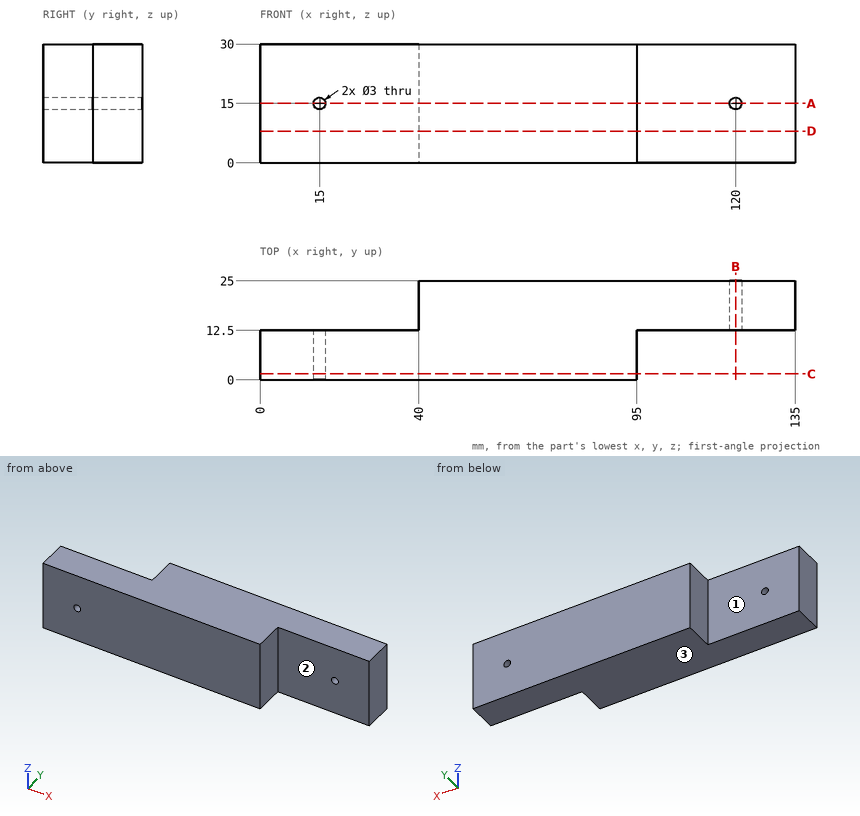
Check sheet for the drawn part. Datum: minimum x, y, z corner. Units: mm. A direction names the side the tool comes from. Round coordinates to 2 decimals unless told otherwise and drop trailing zeros. Order: outer loops, then holes, each group sorted by start corner. A loop starts at its lowest first (then second) coordinate and runs counter-clockwise, first axis right, second up.
1) Tool access check on the marked faces 1, 2 and 3. Record the directions out of +Z, -Z, +X, -X, +Y, -Y that give a thin tool (end or side, any length) a straight path to the whole face; none if there is none.
2) Scan lines: line 1 (X direction, y = 6.5, z = 15); line 2 (Z direction, x = 15, y = 4); line 3 (X direction, y = 20, z = 10). Record each from-to range of solid material in increasing order.
3) Section check A-A (z = 15). Record the boundary of the cut face in (x, y), and give its area (3 significant figures).
4) Go/stop test with flat-tipped pins: pin 1 Ø4 at (y, z) = (6, 22) entering from -X; pin 2 Ø1.8 at (x, z) = (120, 15) entering from -Y; pin 3 Ø4 at (y, z) = (6.5, 14) entering from +X; pin 4 Ø6 at (y, z) = (20, 19.5) entering from -X. Record where each tip stops, or that it passes through.
5) Section check D-D (z = 8). Record the boundary of the cut face in (x, y), and give its area (4 significant figures).
6) Section check B-B (x = 120). Record the boundary of the cut face in (y, z), and give its area (4 significant figures).
7) Section check C-C (y = 1.5). Record the boundary of the cut face in (x, z), and give its area (3 significant figures).
Result:
1. face 1: +Z, -Z, -X, +Y
1. face 2: +Z, -Z, +X, -Y
1. face 3: -Z, +X, -X, +Y, -Y
2. line 1: x = 0 to 13.5, 16.5 to 95
2. line 2: z = 0 to 13.5, 16.5 to 30
2. line 3: x = 40 to 135
3. outline: (0, 0) - (13.5, 0) - (13.5, 12.5) - (0, 12.5) - close; (16.5, 0) - (95, 0) - (95, 12.5) - (118.5, 12.5) - (118.5, 25) - (40, 25) - (40, 12.5) - (16.5, 12.5) - close; (121.5, 12.5) - (135, 12.5) - (135, 25) - (121.5, 25) - close
3. area: 2,300 mm2
4. pin 1: stops at x = 0
4. pin 2: passes through
4. pin 3: stops at x = 95
4. pin 4: stops at x = 40
5. outline: (0, 0) - (95, 0) - (95, 12.5) - (135, 12.5) - (135, 25) - (40, 25) - (40, 12.5) - (0, 12.5) - close
5. area: 2,375 mm2
6. outline: (12.5, 0) - (25, 0) - (25, 13.5) - (12.5, 13.5) - close; (12.5, 16.5) - (25, 16.5) - (25, 30) - (12.5, 30) - close
6. area: 337.5 mm2
7. outline: (0, 0) - (95, 0) - (95, 30) - (0, 30) - close; hole circle Ø3 at (15, 15)
7. area: 2,840 mm2
